Autodesk Inventor part; units mm, degrees
ref_plane "Start Plane" through (0, 0, 0) normal (0, 1, 0) x (-1, 0, 0)
ref_plane "End Plane" through (0, 300, 0) normal (0, 1, 0) x (-1, 0, 0)
ref_plane "YZ Plane" through (0, 0, 0) normal (1, 0, 0) x (0, 1, 0)
ref_plane "Start Plane" through (0, 0, 0) normal (0, 1, 0) x (-1, 0, 0)
ref_plane "End Plane" through (0, 300, 0) normal (0, 1, 0) x (-1, 0, 0)
sketch "Sketch1" plane through (0, 0, 0) normal (0, 1, 0) x (-1, 0, 0)
  line L0 (40, -5) -> (40, 5)
  arc A0 (40, 5) -> (37, 8) centre (37, 5) ccw
  line L1 (37, 8) -> (-37, 8)
  line L2 (14.5, -8) -> (-14.5, -8)
  arc A1 (14.5, -8) -> (16, -6.5) centre (14.5, -6.5) ccw
  line L3 (-25.5, -8) -> (-37, -8)
  arc A2 (-25.5, -8) -> (-24, -6.5) centre (-25.5, -6.5) ccw
  arc A3 (-37, 8) -> (-40, 5) centre (-37, 5) ccw
  line L4 (-40, 5) -> (-40, -5)
  arc A4 (-40, -5) -> (-37, -8) centre (-37, -5) ccw
  line L5 (-24, -6.5) -> (-24, -4.5)
  arc A5 (-24, -4.5) -> (-25, -3.5) centre (-25, -4.5) ccw
  line L6 (-25, -3.5) -> (-29.0014, -3.5)
  arc A6 (-29.8106, -1.9125) -> (-29.0014, -3.5) centre (-29.0014, -2.5) ccw
  arc A7 (-23.7664, 3.9851) -> (-29.8106, -1.9125) centre (-9.58, -16.6) ccw
  arc A8 (-22.9152, 4.25) -> (-23.7664, 3.9851) centre (-22.9152, 2.75) ccw
  line L7 (-22.9152, 4.25) -> (-17.0848, 4.25)
  arc A9 (-16.2336, 3.9851) -> (-17.0848, 4.25) centre (-17.0848, 2.75) ccw
  arc A10 (-10.1894, -1.9125) -> (-16.2336, 3.9851) centre (-30.42, -16.6) ccw
  arc A11 (-10.9986, -3.5) -> (-10.1894, -1.9125) centre (-10.9986, -2.5) ccw
  line L8 (-10.9986, -3.5) -> (-15, -3.5)
  arc A12 (-15, -3.5) -> (-16, -4.5) centre (-15, -4.5) ccw
  line L9 (-16, -4.5) -> (-16, -6.5)
  arc A13 (-16, -6.5) -> (-14.5, -8) centre (-14.5, -6.5) ccw
  line L10 (16, -6.5) -> (16, -4.5)
  arc A14 (16, -4.5) -> (15, -3.5) centre (15, -4.5) ccw
  line L11 (15, -3.5) -> (10.9986, -3.5)
  arc A15 (10.1894, -1.9125) -> (10.9986, -3.5) centre (10.9986, -2.5) ccw
  arc A16 (16.2336, 3.9851) -> (10.1894, -1.9125) centre (30.42, -16.6) ccw
  arc A17 (17.0848, 4.25) -> (16.2336, 3.9851) centre (17.0848, 2.75) ccw
  line L12 (17.0848, 4.25) -> (22.9152, 4.25)
  arc A18 (23.7664, 3.9851) -> (22.9152, 4.25) centre (22.9152, 2.75) ccw
  arc A19 (29.8106, -1.9125) -> (23.7664, 3.9851) centre (9.58, -16.6) ccw
  arc A20 (29.0014, -3.5) -> (29.8106, -1.9125) centre (29.0014, -2.5) ccw
  line L13 (29.0014, -3.5) -> (25, -3.5)
  arc A21 (25, -3.5) -> (24, -4.5) centre (25, -4.5) ccw
  line L14 (1.9858, -3.8) -> (-1.9858, -3.8)
  arc A22 (-2.6929, -3.5071) -> (-1.9858, -3.8) centre (-1.9858, -2.8) ccw
  line L15 (-2.6929, -3.5071) -> (-8.2929, 2.0929)
  arc A23 (-7.5858, 3.8) -> (-8.2929, 2.0929) centre (-7.5858, 2.8) ccw
  line L16 (-7.5858, 3.8) -> (7.5858, 3.8)
  arc A24 (8.2929, 2.0929) -> (7.5858, 3.8) centre (7.5858, 2.8) ccw
  line L17 (8.2929, 2.0929) -> (2.6929, -3.5071)
  arc A25 (1.9858, -3.8) -> (2.6929, -3.5071) centre (1.9858, -2.8) ccw
  circle A26 centre (-34, 0) radius 2.05
  circle A27 centre (34, 0) radius 2.05
  line L18 (25.5, -8) -> (37, -8)
  arc A28 (24, -6.5) -> (25.5, -8) centre (25.5, -6.5) ccw
  arc A29 (37, -8) -> (40, -5) centre (37, -5) ccw
  line L19 (24, -6.5) -> (24, -4.5)
  point P0 (0, 0)
extrude "Body" add sketch "Sketch1" along normal up to surface (300 mm away) from surface at 0
sketch "Sketch2" plane through (0, 0, 0) normal (0, 1, 0) x (-1, 0, 0)
  line L0 (0, 0) -> (10, 0)
ref_plane "Work Plane3" through (0, 0, 0) normal (0, 0, -1) x (-1, 0, 0)
sketch "Sketch3" plane through (0, 0, 0) normal (0, 0, -1) x (-1, 0, 0)
  line L0 (-2, 0) -> (12, 0)
  line L1 (-2, 300) -> (12, 300)
  dimension "d15" = 300
ref_plane "Piano di lavoro4" through (-37, 0, -8) normal (0, 0, 1) x (1, 0, 0)
equation "\"G_OFFSET_START\" = 0"
equation "\"G_OFFSET_END\" = 0"
equation "\"G_L\" = d15"
properties part number "10-081"
For this review, take the finished solid that the model builds, in its own axes (mm). A direction names the side the tool comes from. Round coordinates to 2 decimals unless told otherwise and drop trailing zeros. Order: outer loops, then holes, each group sorted by start corner. A loop starts at its lowest first (then second) coordinate and runs counter-clockwise, first axis right, second up.
Q1. Machinability: for faces 5 (the cylindrical face through (13, 147.9, 1.33)), 6 (the flat face through (20, 148, 4.25)), 7 (the flat face through (31, 148, -8)), which of the approach directions +Z, -Z, +X, -X, +Y, -Y give a long, thin tool a straight path to every point of the face, cutting with its end or side? Answer none if there is none.
Findings below:
face 5: +Y, -Y
face 6: -Z, +Y, -Y
face 7: -Z, +X, -X, +Y, -Y
Q2. Insertion check: P1, Ø6.5, axis at x = -21, y = 221.5, coming from the -Z side; P2, Ø1, axis at y = 149.5, z = -6, coming from the -X side; P3, Ø3, axis at x = 19, y = 109.5, coming from the -Z side; P4, Ø2.5, axis at x = 34, z = 0, coming from the -Y side. Each pin has a flat end and moves straight along its axis. Give the tip position at first contact, or say it passes through.
Findings below:
P1: stops at z = -7.33
P2: stops at x = -39.96
P3: stops at z = 4.25
P4: passes through
Q3. We need section B-B, the plane x = -20. Give the boundary of the cut face in (y, z).
Findings below:
outline: (0, 4.25) - (300, 4.25) - (300, 8) - (0, 8) - close
Q4. Mouldability with a two-part tool opening along X and no side actions: class faces 1 (the cylindrical face through (27.082, 147.9, 1.252)), 2 (the flat face through (-1, 148, 8)), 3 (the flat face through (-40, 148, 0)), 4 (the flat face through (40, 148, 0)) as pulls with the +X half, pulls with the -X half, needs draft (parallel to the pull), parting line crosses it, or undercut.
Findings below:
face 1: undercut
face 2: needs draft
face 3: pulls with the -X half
face 4: pulls with the +X half
Q5. We need section A-A, the plane y = 79. State how many separate pieces and enclosed holes the cut face has, plus the area to 3 significant figures.
Findings below:
separate pieces: 1
enclosed holes: 3
area: 845 mm2
Q6. Wall thickness on line 1 (X direction, y = 252, z = -6.25); line 2 (Z direction, x = 25.5, y = 129.5); line 3 (X direction, y = 80, z = 2.5): over which ranges is each line inside the solid? List them lowest first.
Findings below:
line 1: x = -39.73 to -24, -16 to 16, 24 to 39.73
line 2: z = -8 to -3.5, 2.68 to 8
line 3: x = -40 to -25.71, -14.29 to -8.54, 8.54 to 14.29, 25.71 to 40
